Here's how the part is built. I have some questions about the finished solid (model axes, mm). A direction names the side the tool comes from. Coordinates: 2 decimals unless noted, no trailing zeros. Order: outer loops, then holes, each group sorted by start corner. A loop starts at its lowest first (then second) coordinate and runs counter-clockwise, first axis right, second up. Notation, with made-up numbers: (74.5, 77.5) - (97.5, 77.5) arc R27 ccw to (97.5, 113.5) - close; hole circle Ø10 at (46, -30). An arc over 180 degrees is marked (long way). Answer as CSV lines item,"result". Start each with the question number.
Item 1: I'm going to push flat-ended pins straight in: pin 1 (8.5 mm diameter, centred on y = -16.5, z = 15, fed in from -X) (3 decimals); pin 2 (15.5 mm diameter, centred on x = 25.5, z = 46.5, fed in from -Y); pin 3 (11 mm diameter, centred on y = 1, z = 12.5, fed in from +X) (3 decimals). Where does each tip first touch, or does it pass through?
Item 2: Imagine slicing it at A-A on z = 3. List the corners of the cut face in (x, y) for me (3 decimals).
Item 3: We'd pull the mould along X, two halves only. Please class faces 1 (the face through (61, -21, 42.875)), 2 (the face through (41.275, -1, 4)), 3 (the face through (0, -63.5, 0)), 4 (the face through (-39.365, 61.689, -0.133)): pulls with the +X half, pulls with the -X half, needs draft (parallel to the pull), parting line crosses it, or undercut.
Item 4: Imagine slicing it at B-B on y = -35.5. List the corners of the cut face in (x, z) for me (3 decimals).
Item 5: On a 3-axis mill with a long thin cutter (end or side, diameter ignored), from which of +Z, -Z, +X, -X, +Y, -Y can I reach the whole of each face in a straight line? I mean faces 5 (the face through (39.464, 61.59, 0.133)), 6 (the face through (32.24, 16.55, 51.48)), 7 (the face through (0, 63.5, 0)), 8 (the face through (22.225, -17, 18)), 9 (the face through (84, 0, 38.1)). Say none if no direction works.
Item 6: Imagine slicing it at C-C on x = 65. List the corners of the cut face in (y, z) for me (3 decimals), and give its area (3 significant figures).
Item 7: I need wall thicknesses on line 1 (Z direction, x = -9.5, y = -42.5) (3 decimals); line 2 (X direction, y = 35, z = 1) (3 decimals); line 3 (Y direction, x = 19, z = 31). Which ranges of each line are inside material? Lowest first, please.
from build123d import *

# Parameters (mm, degrees)
F1_DEPTH = 63.5
F0_W     = 23.171081849
F0_H     = 19.05
F2_DEPTH = 25.4
F3_DEPTH = 7.9375
F5_R     = 6.35


with BuildPart() as f1:
    # F0 (on Front) → F1 (new body, symmetric)
    with BuildSketch(Plane.XZ):
        Polygon((22.225, 9.525), (-41.275, 9.525), (-41.275, -9.525), (41.275, -9.525), (41.275, 9.525), align=None)
    extrude(amount=F1_DEPTH, both=True)

    # F0 (on Front) → F2 (join, symmetric)
    with BuildSketch(Plane.XZ):
        with Locations((71.9105409245, 52.4002)):
            Rectangle(F0_W, F0_H)
        with BuildLine():
            Line((22.225, 27.0002), (22.225, 9.525))
            Line((22.225, 9.525), (41.275, 9.525))
            Line((41.275, 9.525), (41.275, 27.0002))
            ThreePointArc((41.275, 27.0002), (45.9246798487, 38.2255201513), (57.15, 42.8752))
            Line((57.15, 42.8752), (60.325, 42.8752))
            Line((60.325, 42.8752), (60.325, 61.9252))
            Line((60.325, 61.9252), (57.15, 61.9252))
            add(Edge.make_bspline(
                [(55.7982156024, 61.8990295497), (56.2487884274, 61.909374971), (56.6993942137, 61.9180941174), (57.15, 61.9252)],
                knots=[110.2855018647, 110.2855018647, 110.2855018647, 110.2855018647, 111.5045361635, 111.5045361635, 111.5045361635, 111.5045361635], degree=3))
            ThreePointArc((55.7982156024, 61.8990295497), (31.9809049121, 51.2132600597), (22.225, 27.0002))
        make_face()
    extrude(amount=F2_DEPTH, both=True)

    # F0 (on Front) → F3 (join, symmetric)
    with BuildSketch(Plane.XZ):
        with BuildLine():
            add(Edge.make_bspline(
                [(-41.275, 9.525), (-25.4582592858, 46.7164983248), (15.0350884427, 60.9630838009), (55.7982156024, 61.8990295497)],
                knots=[0, 0, 0, 0, 110.2855018647, 110.2855018647, 110.2855018647, 110.2855018647], degree=3))
            Line((-41.275, 9.525), (22.225, 9.525))
            Line((22.225, 9.525), (22.225, 27.0002))
            ThreePointArc((22.225, 27.0002), (31.9809049121, 51.2132600597), (55.7982156024, 61.8990295497))
        make_face()
    extrude(amount=F3_DEPTH, both=True)

    # F0 (on Front) → F4 (revolve)
    with BuildSketch(Plane.XZ):
        Polygon((83.496081849, 66.675), (83.496081849, 61.9252), (83.496081849, 42.8752), (83.496081849, 38.1), (111.125, 38.1), (111.125, 66.675), align=None)
    revolve(axis=Axis((83.496081849, 0, 52.3875), (0, 0, 1)))

    # F5
    f5_edges = [f1.edges().sort_by_distance(p)[0] for p in [
        (41.275, -63.5, 0),
        (-41.275, -63.5, 0),
        (41.275, 63.5, 0),
        (-41.275, 63.5, 0),
    ]]
    fillet(f5_edges, radius=F5_R)


solid = f1.part
Responses:
1,pin 1,"stops at x = 22.225"
1,pin 2,"stops at y = -25.4"
1,pin 3,"stops at x = 41.275"
2,outline,"(-41.275, -57.15) arc R6.35 ccw to (-34.925, -63.5) - (34.925, -63.5) arc R6.35 ccw to (41.275, -57.15) - (41.275, 57.15) arc R6.35 ccw to (34.925, 63.5) - (-34.925, 63.5) arc R6.35 ccw to (-41.275, 57.15) - close"
3,face 1,"undercut"
3,face 2,"pulls with the +X half"
3,face 3,"needs draft"
3,face 4,"pulls with the -X half"
4,outline,"(-41.275, -9.525) - (41.275, -9.525) - (41.275, 9.525) - (-41.275, 9.525) - close"
5,face 5,"+Z, -Z, +X, +Y"
5,face 6,"+Z, -X, +Y"
5,face 7,"+Z, -Z, +X, -X, +Y"
5,face 8,"+Z, -X, -Y"
5,face 9,"-Z, +X, +Y, -Y"
6,outline,"(-25.4, 42.875) - (-20.524, 42.875) - (-20.524, 38.1) - (20.524, 38.1) - (20.524, 42.875) - (25.4, 42.875) - (25.4, 61.925) - (20.524, 61.925) - (20.524, 66.675) - (-20.524, 66.675) - (-20.524, 61.925) - (-25.4, 61.925) - close"
6,area,"1,360 mm^2"
7,line 1,"z = -9.525 to 9.525"
7,line 2,"x = -41.275 to 41.275"
7,line 3,"y = -7.94 to 7.94"
